Verification items for this drawing (mm, ordinates from the low corner). Coordinates: 2 decimals unless noted, no trailing zeros. Loops run counter-clockwise (first coordinate to the right, second up) from the corner with the lowest first, then second, coordinate; pieces in that order, holes last. Notation, with made-up numbers: M -36.5,41.25 L -15.5,41.25 A18 cw -15.5,52.25 Z; hole C 21.5,-22.75 d10. An arc over 180 degrees is marked long. Return JSON: item names as keys, results as strings.
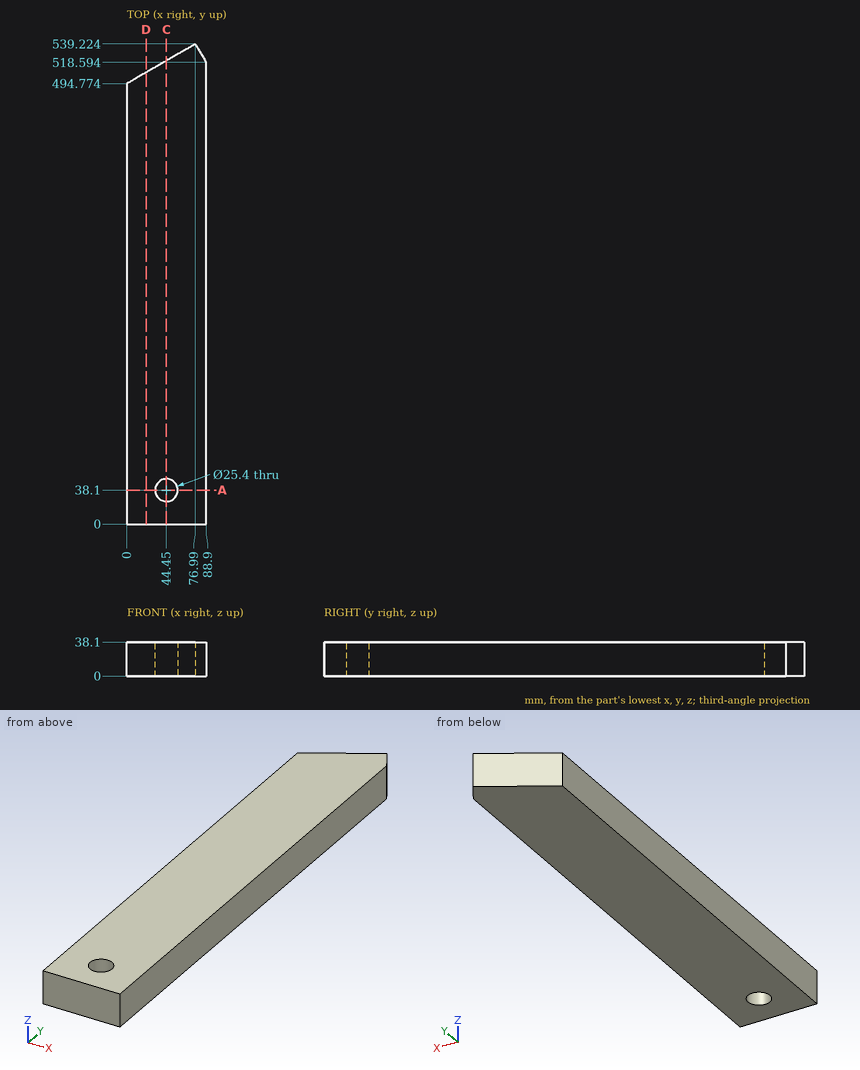
1) Section check C-C on x = 44.45. Record the cut outline in (y, z).
Answers:
{"outline": "M 0,0 L 25.4,0 L 25.4,38.1 L 0,38.1 Z; M 50.8,0 L 520.44,0 L 520.44,38.1 L 50.8,38.1 Z"}
2) Section check D-D on x = 21.5. Record the cut outline in (y, z).
Answers:
{"outline": "M 0,0 L 507.19,0 L 507.19,38.1 L 0,38.1 Z"}
3) Section check A-A on y = 38.1. Record the cut outline in (x, z).
Answers:
{"outline": "M 0,0 L 31.75,0 L 31.75,38.1 L 0,38.1 Z; M 57.15,0 L 88.9,0 L 88.9,38.1 L 57.15,38.1 Z"}
4) Go/stop test with flat-tipped pins: pin 1 Ø23 at (x, y) = (44.45, 38.1) entering from -Z; pin 2 Ø3 at (x, z) = (35.5, 31) entering from +Y (1 decimal). Record where each tip stops, or that it passes through.
Answers:
{"pin 1": "through", "pin 2": "y = 516.1"}
5) Scan lines: line 1 along X through (y, z) = (38, 8); line 2 along Y through (x, z) = (44.45, 28) (1 decimal); line 3 along Y through (x, z) = (44, 14). Record each from-to range of solid material in increasing order. Write a range as [from, to].
Answers:
{"line 1": "[0, 31.75], [57.15, 88.9]", "line 2": "[0, 25.4], [50.8, 520.4]", "line 3": "[0, 25.41], [50.79, 520.18]"}
